Read the model definition and answer for the solid it produces. Units are mm, in the model's axes. A direction names the side the tool comes from. Round coordinates to 2 decimals unless told otherwise and drop trailing zeros. Order: outer loops, then holes, each group sorted by start corner. A loop starts at its lowest first (then second) coordinate and runs counter-clockwise, first axis right, second up. Notation, with made-up numbers: (60.25, 54.5) - (84.25, 54.5) arc R28 cw to (84.25, 80.5) - close; hole circle Ø4 at (37.25, 28.5). An arc over 180 degrees is marked (long way). Answer as a JSON object with one key per item and string values. Group by question number.
Q1. Consider line 1 (Y direction, x = 0, z = 1.25); line 2 (Y direction, x = 39, z = 14.75); line 3 (X direction, y = 19, z = 6.25). Determine where each line is inside the solid, lowest interval first.
Q2. Given pin 1 Ø17 at (x, y) = (5, 8) entering from +Z; pin 2 Ø12 at (x, y) = (-22.5, -27) entering from -Z; pin 3 Ø2 at (x, y) = (32.5, -3) entering from -Z; pin 4 Ø6 at (x, z) = (27.5, 7) entering from -Y, each flat-ended and moving along its own axis, determine where each tip first touches the part or whether it passes through.
Q3. A cutting plane is placed at C-C on y = 31. Determine the outline of the cut face in (x, z).
Q4. A cutting plane is placed at D-D on x = -22. Determine the outline of the cut face in (y, z).
Q5. A cutting plane is placed at A-A on x = 0. Determine the outline of the cut face in (y, z).
Q6. The mould has two halves that part along X. Classify faces 5 (the cylindrical face through (39.85, -3.44, 6.59)), 6 (the cylindrical face through (-22.903, -32.794, 6.591)), 7 (the flat face through (-15, 31, 13)): pulls with the +X half, pulls with the -X half, needs draft (parallel to the pull), parting line crosses it, or undercut.
Q7. A cutting plane is placed at B-B on z = 11.5. Determine the outline of the cut face in (x, y).
Q8. A tool of negligible diameter and unlimited length cuts with its end or side. For faces 1 (the flat face through (-6, 13, 0)), 2 (the flat face through (-20, -29, 13)), 3 (the flat face through (32.757, -5.776, 13.646)), 4 (the conical face through (23.322, -2.012, 6.409)), from which of +Z, -Z, +X, -X, +Y, -Y can it reach the whole face along a straight path? Write none if from no direction.
```python
from build123d import *

# Parameters (mm, degrees)
SKETCH_R           = 17
SKETCH_R_2         = 14
PAD_DEPTH          = 3.5
REVOLUTION_ANGLE   = -10
POLARPATTERN_COUNT = 3


with BuildPart() as part:
    # Sketch → Pad (new body)
    with BuildSketch(Plane.XY):
        Circle(SKETCH_R)
        Circle(SKETCH_R_2, mode=Mode.SUBTRACT)
    extrude(amount=PAD_DEPTH)

    # Sketch001 → Revolution (revolve)
    with BuildSketch(Plane.XZ):
        Polygon((17, 2), (30, 15), (42, 15), (42, 0), (40, 0), (40, 13), (30, 13), (17, 0), align=None)
    revolution = revolve(axis=Axis((0, 0, 0), (0, 0, 1)), revolution_arc=REVOLUTION_ANGLE)

    # PolarPattern: Revolution ×3 about axis
    polarpattern_axis = Axis((0, 0, 0), (0, 0, 1))
    for i in range(1, POLARPATTERN_COUNT):
        add(revolution.rotate(polarpattern_axis, i * 360 / POLARPATTERN_COUNT))


solid = part.part
```
Result set:
{
 "1": {"line 1": "y = -17 to -14, 14 to 17", "line 2": "y = -6.88 to 0", "line 3": "x = -10.97 to -9.52"},
 "2": {"pin 1": "stops at z = 3.5", "pin 2": "stops at z = 0", "pin 3": "stops at z = 13", "pin 4": "stops at y = -4.65"},
 "3": {"outline": "(-17.9, 13) - (-11.28, 13) - (-11.28, 15) - (-17.9, 15) - close"},
 "4": {"outline": "(-35.78, 0) - (-33.41, 0) - (-33.41, 13) - (-26.22, 13) - (-26.22, 15) - (-35.78, 15) - close"},
 "5": {"outline": "(-17, 0) - (-14, 0) - (-14, 3.5) - (-17, 3.5) - close; (14, 0) - (17, 0) - (17, 3.5) - (14, 3.5) - close"},
 "6": {"face 5": "undercut", "face 6": "pulls with the +X half", "face 7": "needs draft"},
 "7": {"outline": "(-27, -32.17) arc R42 ccw to (-21, -36.37) - (-20, -34.64) arc R40 cw to (-25.71, -30.64) - close; (-21, 36.37) - (-20, 34.64) arc R40 cw to (-13.68, 37.59) - (-14.36, 39.47) arc R42 ccw to start; (-18.32, -21.83) arc R28.5 ccw to (-14.25, -24.68) - (-13.25, -22.95) arc R26.5 cw to (-17.03, -20.3) - close; (-14.25, 24.68) - (-13.25, 22.95) arc R26.5 cw to (-9.06, 24.9) - (-9.75, 26.78) arc R28.5 ccw to start; (26.1, -4.6) - (28.07, -4.95) arc R28.5 ccw to (28.5, 0) - (26.5, 0) arc R26.5 cw to start; (39.39, -6.95) - (41.36, -7.29) arc R42 ccw to (42, 0) - (40, 0) arc R40 cw to start"},
 "8": {"face 1": "-Z, +X, -X, +Y, -Y", "face 2": "-Z", "face 3": "+Z, -Z, -Y", "face 4": "-Z, -Y"}
}
